Autodesk Inventor part; units mm, degrees
ref_plane "YZ Plane" through (0, 0, 0) normal (1, 0, 0) x (0, 1, 0)
ref_plane "XZ Plane" through (0, 0, 0) normal (0, 1, 0) x (-1, 0, 0)
ref_plane "XY Plane" through (0, 0, 0) normal (0, 0, 1) x (1, 0, 0)
sketch "Sketch1" plane through (0, 0, 0) normal (0, 0, 1) x (1, 0, 0)
  arc A0 (670.9948, -199.4141) -> (0, 0) centre (254.9219, -370.8299) ccw
  arc A1 (657.7848, -239.4141) -> (30, 0) centre (229.3296, -420.1103) ccw
  arc A2 (657.7848, -239.4141) -> (670.9948, -199.4141) centre (0, 0) ccw
  line L0 (0, 0) -> (30, 0)
  line L1 (657.7848, -239.4141) -> (0, 0)
  line L2 (-143.7228, 0) -> (862.3369, 0)
  point P0 (0, 0)
  dimension "d1" = 30
  dimension "d2" = 40
  dimension "d4" = 20
  dimension "d5" = 465
  dimension "d6" = 450
  dimension "d22" = 700
extrude "Extrusion1" add sketch "Sketch1" along normal blind 4 contours A2 A1 L2 A0 | L2 A1 L0 A0
sketch "Sketch2" plane through (0, 0, 4) normal (0, 0, 1) x (1, 0, 0)
  arc A0 (670.9948, -199.4141) -> (0, 0) centre (254.9219, -370.8299) ccw
  arc A1 (87.1309, 22.5434) -> (74.166, 50.9844) centre (0, 0) ccw
  line L0 (74.166, 50.9844) -> (0, 0)
  line L1 (0, 0) -> (87.1309, 22.5434)
  line L2 (0, 0) -> (30, 0)
  point P0 (78.8927, 43.3122)
  point P1 (0, 0)
  point P2 (0, 0)
  dimension "d9" = 90
  dimension "d16" = 20
extrude "Extrusion2" add sketch "Sketch2" against normal blind 4
sketch "Sketch4" plane through (0, 0, 4) normal (0, 0, 1) x (1, 0, 0)
  line L0 (86.0304, 22.2587) -> (87.1309, 22.5434)
  line L1 (74.166, 50.9844) -> (0, 0)
  line L2 (87.1309, 22.5434) -> (0, 0)
  line L3 (0, 0) -> (30, 0)
  arc A0 (86.0304, 22.2587) -> (30, 0) centre (229.3296, -420.1103) ccw
  line L4 (30, 0) -> (86.0304, 22.2587)
  point P0 (86.0304, 22.2587)
extrude "Extrusion4" cut sketch "Sketch4" against normal blind 10 contours A0 L3 L2
sketch "Sketch5" plane through (0, 0, 4) normal (0, 0, 1) x (1, 0, 0)
  line L0 (0, 0) -> (8.2407, 5.6649)
  line L1 (74.166, 50.9844) -> (0, 0)
  line L2 (0, 0) -> (87.1309, 22.5434)
  line L3 (9.6812, 2.5048) -> (0, 0)
  arc A0 (9.6812, 2.5048) -> (8.2407, 5.6649) centre (0, 0) ccw
  point P0 (9.6812, 2.5048)
  dimension "d21" = 10
extrude "Extrusion5" cut sketch "Sketch5" against normal blind 10
sketch "Sketch6" plane through (0, 0, 4) normal (0, 0, 1) x (1, 0, 0)
  arc A0 (670.9948, -199.4141) -> (78.8927, 43.3122) centre (254.9219, -370.8299) ccw
  arc A1 (258.8056, -24.8926) -> (214.2573, 147.2882) centre (0, 0) ccw
  line L0 (0, 0) -> (214.2573, 147.2882)
  line L1 (0, 0) -> (258.8056, -24.8926)
  line L2 (74.166, 50.9844) -> (8.2407, 5.6649)
  dimension "d23" = 40
  dimension "d24" = 260
extrude "Extrusion6" cut sketch "Sketch6" against normal blind 10
sketch "Sketch7" plane through (0, 0, 4) normal (0, 0, 1) x (1, 0, 0)
  line L0 (0, 0) -> (260.1676, 72.1998)
  line L1 (0, 0) -> (264.5703, 53.8755)
  line L2 (-134.199, 0) -> (805.1938, 0)
  circle A0 centre (260.1676, 72.1998) radius 1.5
  circle A1 centre (264.5703, 53.8755) radius 1.5
  circle A2 centre (281.223, 70.1761) radius 1.5
  circle A3 centre (285.6257, 51.8518) radius 1.5
  line L3 (281.223, 70.1761) -> (285.6257, 51.8518)
  line L4 (285.6257, 51.8518) -> (264.5703, 53.8755)
  line L5 (264.5703, 53.8755) -> (260.1676, 72.1998)
  line L6 (281.223, 70.1761) -> (260.1676, 72.1998)
  dimension "d27" = 15.51
  dimension "d28" = 4
  dimension "d29" = 270
  dimension "d30" = 270
  dimension "d31" = 3
  dimension "d32" = 3
  dimension "d33" = 3
  dimension "d34" = 3
  dimension "d35" = 109
  dimension "d36" = 20
extrude "Extrusion7" cut sketch "Sketch7" against normal through all contours A0 L6 L0 | L0 L5 A0 | A1 L5 L1 | L1 L4 A1 | L6 A0 L5 | L5 A1 L4 | L4 L3 A3 | A3 L3 L4 | L6 L3 A2 | A2 L3 L6
properties part number "spoke4"
Work out the finished part from the listing and answer in its coordinate system (mm). Coordinates: 2 decimals unless noted, no trailing zeros. Write each loop counter-clockwise with the first axis right and the second up, starting at its lowest first coordinate (ties: lowest second). Pieces come first, ordered by that corner, then holes. Notation, with made-up numbers: M -20.5,48.5 L 23.5,48.5 A11 cw 23.5,56.5 Z; hole C 86,46 d9. An arc over 180 degrees is marked long. Use one line per item in the form item = value. Start each with the question number.
1. The part is cut by section C-C (y = -50). Give the vertices of the cut face in (x, z).
2. The part is cut by section A-A (z = 2.3). Give the vertices of the cut face in (x, y), plus the area to 3 significant figures.
3. Each of these flat-tipped pins is pushed along its axis until it touches: P1, Ø1, axis at y = 46.5, z = 2, coming from the -X side; P2, Ø1.5, axis at x = 621.5, z = 1.5, coming from the +Y side; P3, Ø1, axis at x = 602.5, z = 1, coming from the -Y side. Where does it stop, or does it pass through?
4. Straight lines are drawn through the part: probe 1 along X at (y, z) = (-34.5, 0.85); probe 2 along Y at (x, z) = (421.5, 0.4); probe 3 along Y at (x, z) = (332.5, 2.55). For each, find the intervals that lie inside material, in ascending order. Write a range as from..to.
5. The part is cut by section B-B (x = 320). Give the vertices of the cut face in (y, z), plus the area to 3 significant figures.
Evaluation:
q1.outline = M 510.83,0 L 570.47,0 L 570.47,4 L 510.83,4 Z
q2.outline = M 247.67,79.11 A260 cw 256.23,44.11 A465 cw 657.78,-239.41 A700.04 ccw 670.99,-199.41 A450 ccw Z; hole C 260.17,72.2 d3; hole C 264.57,53.88 d3; hole C 281.22,70.18 d3; hole C 285.63,51.85 d3
q2.area = 19,600 mm^2
q3.P1 = 255.72
q3.P2 = -108.78
q3.P3 = -143.35
q4.probe_1 = 489.19..553.89
q4.probe_2 = 3.32..47.2
q4.probe_3 = 33.3..72.43
q5.outline = M 35.96,0 L 74.44,0 L 74.44,4 L 35.96,4 Z
q5.area = 154 mm^2
